Design review of the part shown in the three views and the two pictorial views. Dimensions are in mm from the part's minimum x, y and z. A direction names the side the tool comes from. Coordinates: 2 decimals unless noted, no trailing zeros. Loops run counter-clockwise (first coordinate to the right, second up) from the corner with the lowest first, then second, coordinate; pieces in that order, holes last. Notation, with made-up numbers: (12.5, 45.5) -> (67.5, 45.5) arc R12 ccw to (67.5, 62.5) -> close; hole circle Ø7 at (-14, 37). An arc over 180 degrees is marked (long way). Answer in a Markdown table with one row per item.
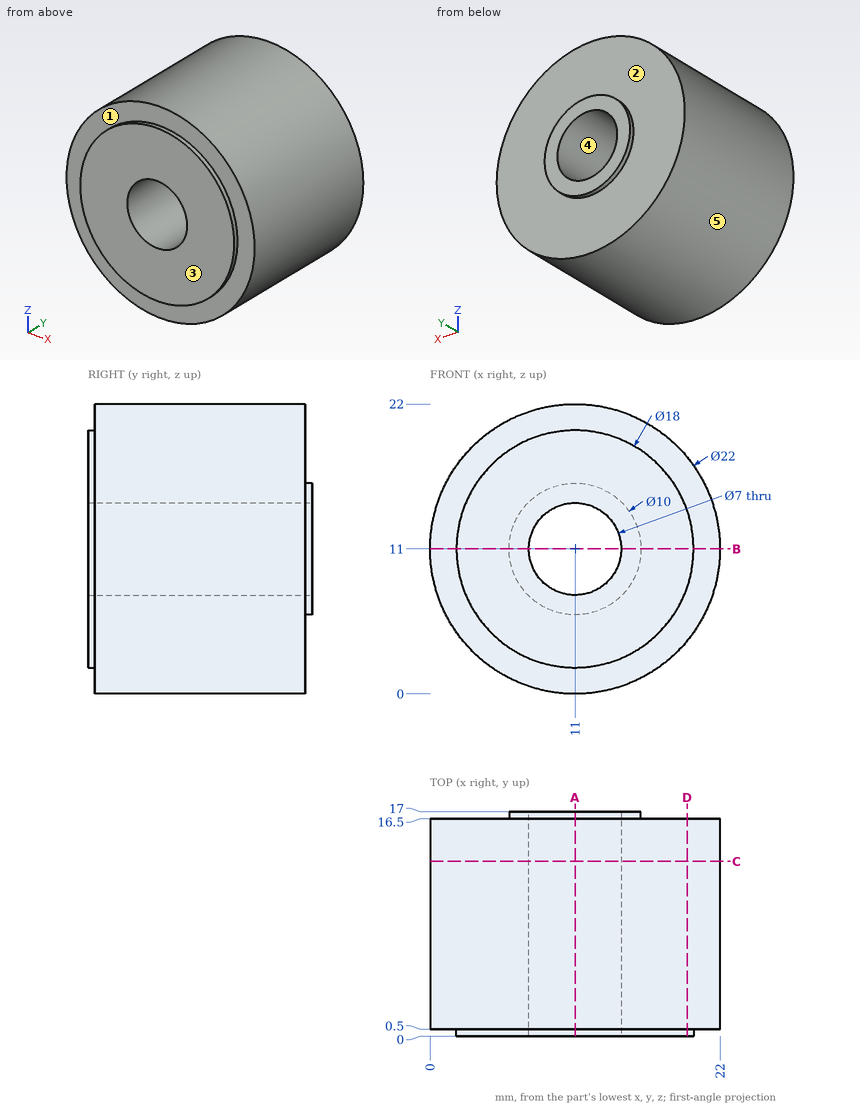
(1) Draft analysis for pull direction X (two halves, no side actions). For the marked faces 3, 4 and 5, state which applies: pulls with the +X half, pulls with the -X half, needs draft (parallel to the pull), parting line crosses it, or undercut.
Evaluation:
| item | result |
|---|---|
| face 3 | needs draft |
| face 4 | undercut |
| face 5 | parting line crosses it |
(2) Take a section at D-D on x = 19.5. Give the boundary of the cut face in (y, z), and give its area (3 significant figures).
Evaluation:
| item | result |
|---|---|
| outline | (0, 8.04) -> (0.5, 8.04) -> (0.5, 4.02) -> (16.5, 4.02) -> (16.5, 17.98) -> (0.5, 17.98) -> (0.5, 13.96) -> (0, 13.96) -> close |
| area | 226 mm² |
(3) To check wall thickness, follow probe 1 along Z at (x, y) = (11, 4); probe 2 along Y at (x, z) = (9.5, 16). State the ranges of each line that lie inside material, in increasing order.
Evaluation:
| item | result |
|---|---|
| probe 1 | z = 0 to 7.5, 14.5 to 22 |
| probe 2 | y = 0 to 16.5 |
(4) Take a section at C-C on y = 13.25. Give the boundary of the cut face in (x, z).
Evaluation:
| item | result |
|---|---|
| outline | circle Ø22 at (11, 11); hole circle Ø7 at (11, 11) |
(5) Take a section at A-A on x = 11. Give the boundary of the cut face in (y, z).
Evaluation:
| item | result |
|---|---|
| outline | (0, 2) -> (0.5, 2) -> (0.5, 0) -> (16.5, 0) -> (16.5, 6) -> (17, 6) -> (17, 7.5) -> (0, 7.5) -> close; (0, 14.5) -> (17, 14.5) -> (17, 16) -> (16.5, 16) -> (16.5, 22) -> (0.5, 22) -> (0.5, 20) -> (0, 20) -> close |
(6) For pin 1 (4 mm diameter, centred on x = 15.5, y = 12.5, fed in from -Z); pin 2 (6 mm diameter, centred on x = 4, y = 3, fed in from +Z); pin 3 (1.5 mm diameter, centred on x = 8.5, y = 6, fed in from -Z), all flat-tipped, find the tip position at first contact; note any pin that passes through.
Evaluation:
| item | result |
|---|---|
| pin 1 | stops at z = 0.29 |
| pin 2 | stops at z = 21.25 |
| pin 3 | stops at z = 0.14 |
(7) Tool access review of the marked faces 1 and 2: name each direction out of +Z, -Z, +X, -X, +Y, -Y from which nothing blocks a thin tool from reaching the whole face with its end or side.
Evaluation:
| item | result |
|---|---|
| face 1 | -Y |
| face 2 | +Y |
(8) Take a section at B-B on z = 11. Give the boundary of the cut face in (x, y).
Evaluation:
| item | result |
|---|---|
| outline | (0, 0.5) -> (2, 0.5) -> (2, 0) -> (7.5, 0) -> (7.5, 17) -> (6, 17) -> (6, 16.5) -> (0, 16.5) -> close; (14.5, 0) -> (20, 0) -> (20, 0.5) -> (22, 0.5) -> (22, 16.5) -> (16, 16.5) -> (16, 17) -> (14.5, 17) -> close |
